Source: CAD feature listing. Evaluate the final solid. Frame: model axes, mm. A direction names the side the tool comes from. Give positions to 0.01 mm unless a question says otherwise; leave off trailing zeros. Loops run counter-clockwise (first coordinate to the right, second up) from the corner with the lowest first, then second, coordinate; pieces in that order, holes last. Notation, with made-up numbers: M -4,-19 L 21,-19 A21 cw 21,-2 Z; hole C 63,60.25 d11. An arc over 180 degrees is marked long. Write item = value, one per line.
from build123d import *

# Parameters (mm, degrees)
SKETCH2_R           = 12.5
BOSS_EXTRUDE1_DEPTH = 12.72
CHAMFER1_SIZE       = 1
BOSS_EXTRUDE2_DEPTH = 18


with BuildPart() as part:
    # Sketch1 → Revolve1 (revolve)
    with BuildSketch(Plane(origin=(0, 0, 0), x_dir=(0, 0, -1), z_dir=(1, 0, 0))):
        Polygon((0, 104.5), (0, -104.5), (-19.925, -104.5), (-21.965, -98.5), (-35, -98.5), (-35, -94.5), (-39.9, -94.5), (-39.9, -80.5), (-40, -80.5), (-40, 89.5), (-39.9, 89.5), (-39.9, 104.5), align=None)
    revolve(axis=Axis((0, 104.5, 0), (0, -1, 0)))

    # Sketch2 → Boss-Extrude1 (add)
    with BuildSketch(Plane.XZ.offset(104.5)):
        with Locations(Location((0, 0, 0), (0, 0, 90))):
            Circle(SKETCH2_R)
    extrude(amount=BOSS_EXTRUDE1_DEPTH)

    # Chamfer1
    chamfer1_edges = [part.edges().sort_by_distance(p)[0] for p in [
        (0, -98.5, -35),
        (0, -94.5, -39.9),
        (0, 104.5, -39.9),
    ]]
    chamfer(chamfer1_edges, length=CHAMFER1_SIZE)

    # Sketch3 → Boss-Extrude2 (add)
    with BuildSketch(Plane.XZ.offset(117.22)):
        Polygon((0, 16.310145105), (-14.125, 8.155072552), (-14.125, -8.155072552), (0, -16.310145105), (14.125, -8.155072552), (14.125, 8.155072552), align=None)
    extrude(amount=BOSS_EXTRUDE2_DEPTH)

    # Sketch4 → Revolve2 (revolve)
    with BuildSketch(Plane(origin=(0, 0, 0), x_dir=(0, 0, -1), z_dir=(1, 0, 0)), mode=Mode.PRIVATE) as revolve2_sk:
        Polygon((-6, -135.22), (-6, -139.22), (-8, -139.22), (-12, -135.22), align=None)
    revolve(revolve2_sk.sketch.rotate(Axis((0, 258.155027854, 0), (0, -1, 0)), 180), axis=Axis((0, 258.155027854, 0), (0, -1, 0)))

    # Sketch6 → Revolve3 (revolve)
    with BuildSketch(Plane(origin=(21.67, 0, 0), x_dir=(0, 0, -1), z_dir=(1, 0, 0))):
        Polygon((20.45, 104.5), (24.3, 104.5), (24.3, 107.26), (25.275, 107.26), (25.275, 113.02), (24.54, 113.02), (23.56, 117.19), (21.355, 117.19), (21.11, 120.5), (20.45, 120.5), align=None)
    revolve3 = revolve(axis=Axis((21.67, 104.5, -18.45), (0, 1, 0)))

    # Mirror1: Revolve3 across plane
    add(revolve3.mirror(Plane.XY))


solid = part.part
1. Material intervals for probe 1 along Z at (x, y) = (21.67, 109.75) (3 decimals); probe 2 along Y at (x, z) = (-13.5, 1); probe 3 along X at (y, z) = (110.75, -18.45) (3 decimals), sorted ascending. Write a range as from..to.
Derived:
probe_1 = -25.275..-20.45, -16.45..-11.625, 11.625..16.45, 20.45..25.275
probe_2 = -135.22..-117.22, -104.5..104.5
probe_3 = 14.845..19.67, 23.67..28.495
2. Reachability of faces 4 (the flat face through (6.96, -126.09, -12.29)), 5 (the cylindrical face through (21, -96, -28)), 6 (the flat face through (-7.161, -126.094, -12.176)), 7 (the flat face through (7.161, -126.094, 12.176)) from +Z, -Z, +X, -X, +Y, -Y: full face, straight path, thin tool, end or side. Return the list, or none.
Derived:
face_4 = -Z, +X, -Y
face_5 = -Y
face_6 = -Z, -X, -Y
face_7 = +Z, +X, -Y
3. First-contact query: pin 1 Ø8 at (x, z) = (17.5, -3) entering from -Y; pin 2 Ø10 at (y, z) = (71.5, 4) entering from +X; pin 3 Ø1.2 at (x, z) = (21, 19) entering from +Y. Flat tips, straight axial feed; report the tip coordinate or a pass-through.
Derived:
pin_1 = -135.22
pin_2 = 40
pin_3 = 104.5
4. Cut plane A-A, the plane y = 25.5. Return the cut outline in (x, z).
Derived:
outline = C 0,0 d80
5. Pull-direction query (Z, two-part tool) for faces 1 (the conical face through (16.45, 116.52, 17.76)), 2 (the flat face through (-6.96, -126.09, 12.29)), 3 (the flat face through (6, -139.22, -2)); classes: +Z half, -Z half, draft (parallel to the pull), parting line (faces both ways), or undercut.
Derived:
face_1 = undercut
face_2 = +Z half
face_3 = draft
